Source: CAD feature listing. Evaluate the final solid. Frame: model axes, mm. A direction names the side the tool comes from. Round coordinates to 2 decimals unless told otherwise and drop trailing zeros. Order: outer loops, then holes, each group sorted by start corner. A loop starts at its lowest first (then second) coordinate and runs counter-clockwise, first axis right, second up. Notation, with made-up numbers: (-25, 63.5) - (-20, 63.5) arc R34 ccw to (-20, 99.5) - close; hole circle Ø3 at (13.5, -8.5). An arc over 180 degrees is marked (long way). Put each result on its own line as item: value. Start each with the question number.
1) Mould query, pull axis Y, two halves, no side actions, for faces 1 (the face through (-2, 6, 35)), 2 (the face through (-27.5, 0, 20)), 3 (the face through (0, -20, 6)). Classes: +Y half, -Y half, draft (parallel to the pull), parting line (faces both ways), or undercut.
2) Line query: probe 1 along Y at (x, z) = (-24.4, 14); probe 2 along X at (y, z) = (18, 38); probe 3 along X at (y, z) = (-5.5, 12). Output: solid intervals per line, ascending. Write a range as [from, to].
3) Section C-C on x = 0. Output: boundary loops of the cut face in (y, z), then the cut area to 3 significant figures.
4) Section D-D on x = -15. Output: boundary loops of the cut face in (y, z).
5) Contact query for flat-ended pins moving along their axis: P1, Ø15.5, axis at x = 0, y = 0, coming from the -Z side; P2, Ø3, axis at x = 15, y = -15, coming from the +Z side; P3, Ø4, axis at x = -3.5, z = 35.5, coming from the -Y side; P4, Ø3, axis at x = 2.5, z = 12, coming from the -Y side. Output: stop coordinate, or through.
6) Section A-A on z = 14. State how many separate pieces and enclosed holes the cut face has, then the cut area to 3 significant figures.
7) Access query for faces 4 (the face through (6, 0, 17)), 5 (the face through (17, -2, 25)), 6 (the face through (-8.3, 0.1, 40)), 7 (the face through (17, 2, 25)), 8 (the face through (-1.73, -7.81, 37.53)). Directions: +Z, -Z, +X, -X, +Y, -Y. A direction counts if a zero-diameter tool reaches every point of the face in a straight line with its end or side. Return the directions, or none.
```python
from build123d import *

# Parameters (mm, degrees)
SKETCH1_W           = 45
SKETCH1_H           = 40
BOSS_EXTRUDE1_DEPTH = 10
SKETCH2_W           = 5
SKETCH2_H           = 40
BOSS_EXTRUDE2_DEPTH = 40
SKETCH3_R           = 12.5
BOSS_EXTRUDE3_DEPTH = 30
SKETCH4_R           = 6
CUT_EXTRUDE1_DEPTH  = 53.5
SKETCH5_R           = 8
CUT_EXTRUDE2_DEPTH  = 5
SKETCH6_R           = 1.75
CUT_EXTRUDE3_DEPTH  = 53.5
SKETCH7_W           = 11
SKETCH7_H           = 4
BOSS_EXTRUDE4_DEPTH = 30
SKETCH8_R           = 1.75
CUT_EXTRUDE4_DEPTH  = 71.887234394


with BuildPart() as part:
    # Sketch1 → Boss-Extrude1 (new body)
    with BuildSketch(Plane.XY):
        Rectangle(SKETCH1_W, SKETCH1_H)
    extrude(amount=BOSS_EXTRUDE1_DEPTH)

    # Sketch2 → Boss-Extrude2 (add)
    with BuildSketch(Plane.XY):
        with Locations((-25, 0)):
            Rectangle(SKETCH2_W, SKETCH2_H)
        with Locations((25, 0)):
            Rectangle(SKETCH2_W, SKETCH2_H)
    extrude(amount=BOSS_EXTRUDE2_DEPTH)

    # Sketch3 → Boss-Extrude3 (add)
    with BuildSketch(Plane.XY.offset(10)):
        Circle(SKETCH3_R)
    extrude(amount=BOSS_EXTRUDE3_DEPTH)

    # Sketch4 → Cut-Extrude1 (cut, through all)
    with BuildSketch(Plane(origin=(0, 0, 0), x_dir=(-1, 0, 0), z_dir=(0, 0, -1))):
        Circle(SKETCH4_R)
    extrude(amount=-CUT_EXTRUDE1_DEPTH, mode=Mode.SUBTRACT)

    # Sketch5 → Cut-Extrude2 (cut)
    with BuildSketch(Plane.XY.offset(40)):
        Circle(SKETCH5_R)
    extrude(amount=-CUT_EXTRUDE2_DEPTH, mode=Mode.SUBTRACT)

    # Sketch6 → Cut-Extrude3 (cut, through all)
    with BuildSketch(Plane(origin=(0, 0, 0), x_dir=(-1, 0, 0), z_dir=(0, 0, -1))):
        with Locations((-15, 15)):
            Circle(SKETCH6_R)
        with Locations((15, 15)):
            Circle(SKETCH6_R)
        with Locations((15, -15)):
            Circle(SKETCH6_R)
        with Locations((-15, -15)):
            Circle(SKETCH6_R)
    extrude(amount=-CUT_EXTRUDE3_DEPTH, mode=Mode.SUBTRACT)

    # Sketch7 → Boss-Extrude4 (add)
    with BuildSketch(Plane.XY.offset(10)):
        with Locations((-17, 0)):
            Rectangle(SKETCH7_W, SKETCH7_H)
        with Locations((17, 0)):
            Rectangle(SKETCH7_W, SKETCH7_H)
    extrude(amount=BOSS_EXTRUDE4_DEPTH)

    # Sketch8 → Cut-Extrude4 (cut, through all)
    with BuildSketch(Plane.ZY.offset(27.5)):
        with Locations((35, 15)):
            Circle(SKETCH8_R)
        with Locations(Location((35, -15, 0), (0, 0, 90))):
            Circle(SKETCH8_R)
        with Locations((14, 15)):
            Circle(SKETCH8_R)
        with Locations(Location((14, -15, 0), (0, 0, 90))):
            Circle(SKETCH8_R)
    extrude(amount=-CUT_EXTRUDE4_DEPTH, mode=Mode.SUBTRACT)


solid = part.part
```
Answer sheet:
1. face 1: undercut
1. face 2: draft
1. face 3: -Y half
2. probe 1: [-20, -16.75], [-13.25, 13.25], [16.75, 20]
2. probe 2: [-27.5, -22.5], [22.5, 27.5]
2. probe 3: [-27.5, -22.5], [-11.22, -2.4], [2.4, 11.22], [22.5, 27.5]
3. outline: (-20, 0) - (-6, 0) - (-6, 35) - (-8, 35) - (-8, 40) - (-12.5, 40) - (-12.5, 10) - (-20, 10) - close; (6, 0) - (20, 0) - (20, 10) - (12.5, 10) - (12.5, 40) - (8, 40) - (8, 35) - (6, 35) - close
3. area: 650 mm^2
4. outline: (-20, 0) - (-16.75, 0) - (-16.75, 10) - (-20, 10) - close; (-13.25, 0) - (13.25, 0) - (13.25, 10) - (2, 10) - (2, 40) - (-2, 40) - (-2, 10) - (-13.25, 10) - close; (16.75, 0) - (20, 0) - (20, 10) - (16.75, 10) - close
5. P1: z = 0
5. P2: through
5. P3: y = -12.41
5. P4: y = -12.46
6. separate pieces: 5
6. enclosed holes: 1
6. area: 788 mm^2
7. face 4: +Z, -Z
7. face 5: +Z, -Y
7. face 6: +Z, +X, -X, +Y, -Y
7. face 7: +Z, +Y
7. face 8: +Z
